from build123d import *

# Parameters (mm, degrees)
EXTRUDE_1_DEPTH = 35
SKETCH_2_R      = 14
EXTRUDE_2_DEPTH = 6


with BuildPart() as part:
    # 草图1 → 凸台-拉伸1 (new body)
    with BuildSketch(Plane(origin=(0, 0, 0), x_dir=(1, 0, 0), z_dir=(0, 1, 0))):
        with BuildLine():
            Line((4.582575695, -10), (-4.582575695, -10))
            ThreePointArc((-4.582575695, -10), (-7.778174593, -7.778174593), (-10, -4.582575695))
            Line((-10, -4.582575695), (-10, 4.582575695))
            ThreePointArc((-10, 4.582575695), (-7.778174593, 7.778174593), (-4.582575695, 10))
            Line((-4.582575695, 10), (4.582575695, 10))
            ThreePointArc((4.582575695, 10), (7.778174593, 7.778174593), (10, 4.582575695))
            Line((10, 4.582575695), (10, -4.582575695))
            ThreePointArc((10, -4.582575695), (7.778174593, -7.778174593), (4.582575695, -10))
        make_face()
    extrude(amount=EXTRUDE_1_DEPTH)

    # 草图2 → 凸台-拉伸2 (add)
    with BuildSketch(Plane(origin=(0, 35, 0), x_dir=(1, 0, 0), z_dir=(0, 1, 0))):
        with Locations(Location((0, 0, 0), (0, 0, 270))):
            Circle(SKETCH_2_R)
    extrude(amount=EXTRUDE_2_DEPTH)


solid = part.part
Could you check a few things on this model? Use its own coordinates, in mm. A direction names the side the tool comes from. Give positions to 0.01 mm unless a question says otherwise; leave off trailing zeros. Order: outer loops, then holes, each group sorted by start corner. A loop starts at its lowest first (then second) coordinate and runs counter-clockwise, first axis right, second up. Notation, with made-up numbers: (-6, 62.25) -> (44, 62.25) arc R9 ccw to (44, 76.25) -> close; hole circle Ø9 at (-34.5, 57.25). An arc over 180 degrees is marked (long way). Return JSON: item names as keys, results as strings.
1. Imagine slicing it at B-B on z = 0. List the corners of the cut face in (x, y) for me, then the cut area to 3 significant figures.
Answer list:
{"outline": "(-14, 35) -> (-10, 35) -> (-10, 0) -> (10, 0) -> (10, 35) -> (14, 35) -> (14, 41) -> (-14, 41) -> close", "area": "868 mm2"}
2. Imagine slicing it at C-C on z = 12.25. List the corners of the cut face in (x, y) for me.
Answer list:
{"outline": "(-6.78, 35) -> (6.78, 35) -> (6.78, 41) -> (-6.78, 41) -> close"}
3. On a 3-axis mill with a long thin cutter (end or side, diameter ignored), from which of +Z, -Z, +X, -X, +Y, -Y can I reach the whole of each face in a straight line? I mean faces 1 (the cylindrical face through (7.739, 17.255, -7.817)), 2 (the flat face through (-10, 17, 0)), 3 (the cylindrical face through (7.817, 17.255, 7.739)), 4 (the cylindrical face through (-7.739, 17.255, 7.817)), 5 (the flat face through (0, 17, -10)). Say none if no direction works.
Answer list:
{"face 1": "-Z, +X, -Y", "face 2": "+Z, -Z, -X, -Y", "face 3": "+Z, +X, -Y", "face 4": "+Z, -X, -Y", "face 5": "-Z, +X, -X, -Y"}
4. For pin 1 Ø7.5 at (x, y) = (0, 18.5) entering from -Z; pin 2 Ø3 at (x, y) = (-6.5, 7) entering from +Z; pin 3 Ø4 at (y, z) = (13, 8.5) entering from -X, each with a flat end and sliding along its axis, tell me the tip position at first contact or that it passes through.
Answer list:
{"pin 1": "stops at z = -10", "pin 2": "stops at z = 9.8", "pin 3": "stops at x = -8.87"}
5. Imagine slicing it at D-D on z = -12. List the corners of the cut face in (x, y) for me, then the cut area to 3 significant figures.
Answer list:
{"outline": "(-7.21, 35) -> (7.21, 35) -> (7.21, 41) -> (-7.21, 41) -> close", "area": "86.5 mm2"}
6. I need wall thicknesses on line 1 (Y direction, x = 11, z = 1); line 2 (Z direction, x = -0.25, y = 14); line 3 (Z direction, x = -4, y = 37). Which ranges of each line are inside material? Lowest first, please. Write a range as from..to.
Answer list:
{"line 1": "y = 35..41", "line 2": "z = -10..10", "line 3": "z = -13.42..13.42"}
7. Imagine slicing it at A-A on y = 4.5. List the corners of the cut face in (x, z) for me.
Answer list:
{"outline": "(-10, -4.58) arc R11 ccw to (-4.58, -10) -> (4.58, -10) arc R11 ccw to (10, -4.58) -> (10, 4.58) arc R11 ccw to (4.58, 10) -> (-4.58, 10) arc R11 ccw to (-10, 4.58) -> close"}
